from build123d import *

# Parameters (mm, degrees)
ESQUISSE1_R        = 11.25
ESQUISSE1_R_2      = 3.5
BOSS_EXTRU_1_DEPTH = 5
CONG_1_R           = 5


with BuildPart() as part:
    # Esquisse1 → Boss.-Extru.1 (new body)
    with BuildSketch(Plane.XY):
        Polygon((-40, 0), (40, 0), (40, 40), (12.5, 103), (-12.5, 103), (-40, 40), align=None)
        with Locations((0, 85)):
            Circle(ESQUISSE1_R, mode=Mode.SUBTRACT)
        with Locations((0, 20)):
            Circle(ESQUISSE1_R_2, mode=Mode.SUBTRACT)
        with Locations((30, 20)):
            Circle(ESQUISSE1_R_2, mode=Mode.SUBTRACT)
        with Locations((-30, 20)):
            Circle(ESQUISSE1_R_2, mode=Mode.SUBTRACT)
    extrude(amount=BOSS_EXTRU_1_DEPTH)

    # Congé1
    cong_1_edges = [part.edges().sort_by_distance(p)[0] for p in [
        (-12.5, 103, 2.5),
        (12.5, 103, 2.5),
        (40, 40, 2.5),
        (40, 0, 2.5),
        (-40, 0, 2.5),
        (-40, 40, 2.5),
    ]]
    fillet(cong_1_edges, radius=CONG_1_R)


solid = part.part
Read the model definition and answer for the solid it produces. Units are mm, in the model's axes. Give positions to 0.01 mm unless a question says otherwise; leave off trailing zeros. Loops run counter-clockwise (first coordinate to the right, second up) from the corner with the lowest first, then second, coordinate; pieces in that order, holes last. Notation, with made-up numbers: (23, 75) -> (31, 75) arc R20 cw to (31, 96) -> close; hole circle Ø6 at (18, 76.25). An arc over 180 degrees is marked (long way). Use a Markdown table: item, result.
Q1. Find the intervals of material crossed by line 1 along Y through (x, z) = (0, 1.9); line 2 along Y through (x, z) = (-1.5, 3.2); line 3 along Y through (x, z) = (7.5, 1.9), in increasing order.
Solved:
| item | result |
|---|---|
| line 1 | y = 0 to 16.5, 23.5 to 73.75, 96.25 to 103 |
| line 2 | y = 0 to 16.84, 23.16 to 73.85, 96.15 to 103 |
| line 3 | y = 0 to 76.61, 93.39 to 103 |
Q2. Section D-D, the plane x = 30 is taken. Determine the outline of the cut face in (y, z).
Solved:
| item | result |
|---|---|
| outline | (0, 0) -> (16.5, 0) -> (16.5, 5) -> (0, 5) -> close; (23.5, 0) -> (62.91, 0) -> (62.91, 5) -> (23.5, 5) -> close |
Q3. Section A-A, the plane x = 0 is taken. Determine the outline of the cut face in (y, z), then the cut area to 4 significant figures.
Solved:
| item | result |
|---|---|
| outline | (0, 0) -> (16.5, 0) -> (16.5, 5) -> (0, 5) -> close; (23.5, 0) -> (73.75, 0) -> (73.75, 5) -> (23.5, 5) -> close; (96.25, 0) -> (103, 0) -> (103, 5) -> (96.25, 5) -> close |
| area | 367.5 mm^2 |
Q4. Section C-C, the plane z = 1.95 is taken. Determine the outline of the cut face in (x, y).
Solved:
| item | result |
|---|---|
| outline | (-40, 5) arc R5 ccw to (-35, 0) -> (35, 0) arc R5 ccw to (40, 5) -> (40, 38.96) arc R5 ccw to (39.58, 40.96) -> (13.81, 100) arc R5 ccw to (9.23, 103) -> (-9.23, 103) arc R5 ccw to (-13.81, 100) -> (-39.58, 40.96) arc R5 ccw to (-40, 38.96) -> close; hole circle Ø7 at (-30, 20); hole circle Ø22.5 at (0, 85); hole circle Ø7 at (0, 20); hole circle Ø7 at (30, 20) |
Q5. Determine the mould class of faces 1 (the face through (31.88, 22.95, 2.46)), 2 (the face through (-38, 1, 3)), 3 (the face through (39.9, 39.96, 2.54)) for opening direction Y: pulls with the +Y half, pulls with the -Y half, needs draft (parallel to the pull), parting line crosses it, or undercut.
Solved:
| item | result |
|---|---|
| face 1 | undercut |
| face 2 | pulls with the -Y half |
| face 3 | pulls with the +Y half |
Q6. Each of these flat-tipped pins is pushed along its axis until it touches: pin 1 (11 mm diameter, centred on x = 0, y = 20, fed in from -Z); pin 2 (3 mm diameter, centred on x = 31, z = 2.5, fed in from +Y); pin 3 (5.5 mm diameter, centred on x = 30, y = 20, fed in from +Z); pin 4 (3 mm diameter, centred on x = -27.5, z = 1, fed in from +Y). Where does it stop, or does it pass through?
Solved:
| item | result |
|---|---|
| pin 1 | stops at z = 0 |
| pin 2 | stops at y = 64.05 |
| pin 3 | passes through |
| pin 4 | stops at y = 72.07 |
Q7. Section B-B, the plane y = 20 is taken. Determine the outline of the cut face in (x, z), then the cut area to 3 significant figures.
Solved:
| item | result |
|---|---|
| outline | (-40, 0) -> (-33.5, 0) -> (-33.5, 5) -> (-40, 5) -> close; (-26.5, 0) -> (-3.5, 0) -> (-3.5, 5) -> (-26.5, 5) -> close; (3.5, 0) -> (26.5, 0) -> (26.5, 5) -> (3.5, 5) -> close; (33.5, 0) -> (40, 0) -> (40, 5) -> (33.5, 5) -> close |
| area | 295 mm^2 |
